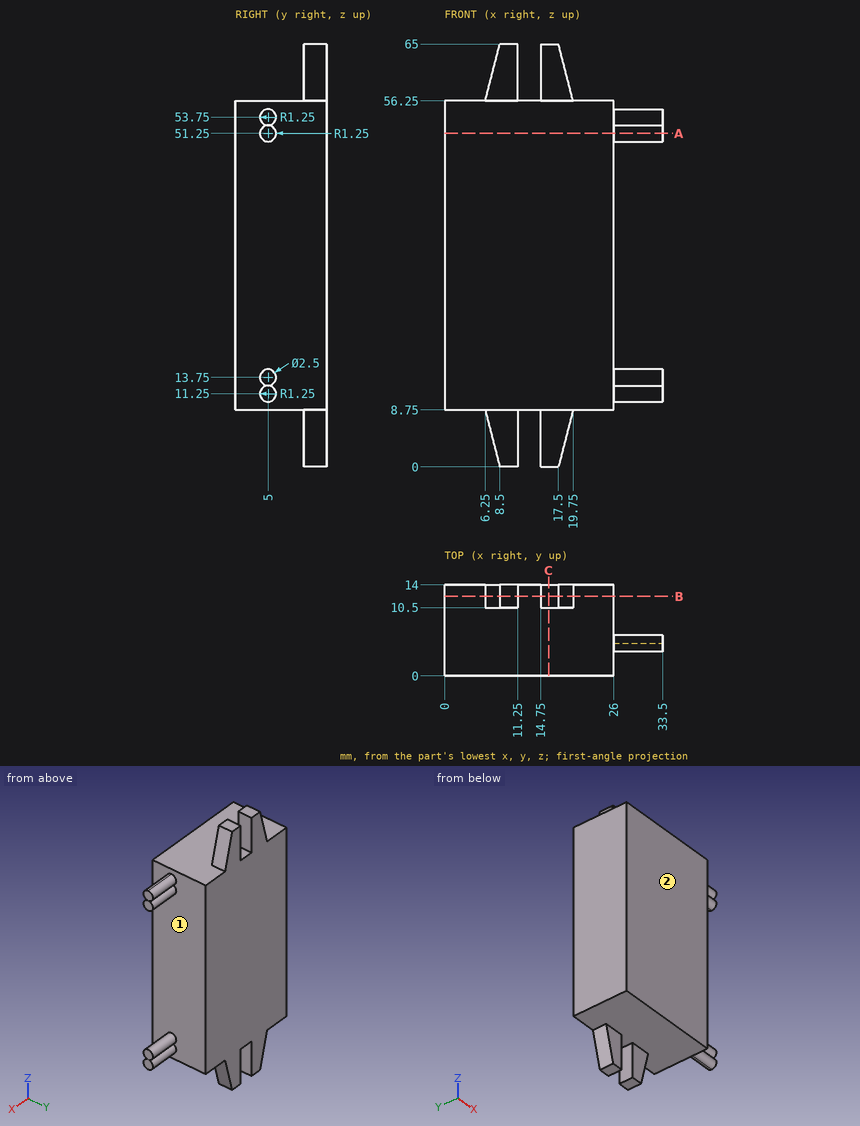
Part print with two shaded views. Sizes in mm from the minimum x, y, z corner. Round coordinates to 2 decimals unless told otherwise and drop trailing zeros. Order: outer loops, then holes, each group sorted by start corner. A loop starts at its lowest first (then second) coordinate and runs counter-clockwise, first axis right, second up. Notation, with made-up numbers: (-6.75, 62.25) -> (40.25, 62.25) arc R23 cw to (40.25, 99.25) -> close; hole circle Ø11 at (-24.5, 25). An arc over 180 degrees is marked (long way). Write each question's results on one line, items separated by ' | '.
1. Flat gauge pins, fed straight in: P1, Ø3, axis at y = 11.5, z = 4, coming from the -X side; P2, Ø2.5, axis at x = 18.5, z = 3.5, coming from the -Y side; P3, Ø2, axis at x = 13.5, y = 4.5, coming from the -Z side. Where does each tip first touch, or does it go through?
Findings below:
P1: stops at x = 7.09 | P2: stops at y = 10.5 | P3: stops at z = 8.75
2. Cut at C-C (x = 16). Give the cut face in (y, z).
Findings below:
outline: (0, 8.75) -> (10.5, 8.75) -> (10.5, 0) -> (14, 0) -> (14, 65) -> (10.5, 65) -> (10.5, 56.25) -> (0, 56.25) -> close
3. Cut at A-A (z = 51.25). Give the cut face in (x, y).
Findings below:
outline: (0, 0) -> (26, 0) -> (26, 3.75) -> (33.5, 3.75) -> (33.5, 6.25) -> (26, 6.25) -> (26, 14) -> (0, 14) -> close
4. Wall check: line 1 along Z through (x, y) = (22, 11.5); line 2 along X through (y, z) = (10.5, 24); line 3 along Y through (x, z) = (18, 8). Give the ranges that are in metal, low to high. Write a range as [from, to].
Findings below:
line 1: z = [8.75, 56.25] | line 2: x = [0, 26] | line 3: y = [10.5, 14]
5. Pull direction Z, two halves, no side cores. Call the marked faces 1 and 2: pulls with the +Z half, pulls with the -Z half, needs draft (parallel to the pull), parting line crosses it, or undercut.
Findings below:
face 1: undercut | face 2: needs draft
6. Cut at B-B (y = 12.25). Give the cut face in (x, z), plus the area to 3 significant figures.
Findings below:
outline: (0, 8.75) -> (6.25, 8.75) -> (8.5, 0) -> (11.25, 0) -> (11.25, 8.75) -> (14.75, 8.75) -> (14.75, 0) -> (17.5, 0) -> (19.75, 8.75) -> (26, 8.75) -> (26, 56.25) -> (19.75, 56.25) -> (17.5, 65) -> (14.75, 65) -> (14.75, 56.25) -> (11.25, 56.25) -> (11.25, 65) -> (8.5, 65) -> (6.25, 56.25) -> (0, 56.25) -> close | area: 1,370 mm²
